The listing builds one solid part. Answer for the finished solid, in the listing's coordinates (mm). A direction names the side the tool comes from. Round coordinates to 2 decimals unless told otherwise and drop trailing zeros. Loops run counter-clockwise (first coordinate to the right, second up) from the corner with the lowest first, then second, coordinate; pieces in that order, holes last. Notation, with made-up numbers: (82.25, 41) -> (137.25, 41) arc R14 cw to (137.25, 56) -> close; hole circle Ø4 at (36, 63.5). An arc over 180 degrees is marked (long way). One line per question, with ' | ' between items.
from build123d import *

# Parameters (mm, degrees)
SKETCH_W             = 70
SKETCH_H             = 40
PAD_DEPTH            = 8.8
POCKET_DEPTH         = 4
SKETCH002_R          = 2
POCKET001_DEPTH      = 4.801
SKETCH003_W          = 64.25
SKETCH003_H          = 24
POCKET002_DEPTH      = 4.8
SKETCH004_R          = 2
POCKET003_DEPTH      = 4
SKETCH005_W          = 35
SKETCH005_H          = 12
POCKET004_DEPTH      = 4
POCKET005_DEPTH      = 8.801
SKETCH009_W          = 5.75
SKETCH009_H          = 15
POCKET006_DEPTH      = 2.3
FILLET_R             = 2.75
CHAMFER_SIZE         = 1
BODY_PLACEMENT_ANGLE = 90


with BuildPart() as part:
    # Sketch → Pad (new body)
    with BuildSketch(Plane.XZ):
        Rectangle(SKETCH_W, SKETCH_H)
    extrude(amount=PAD_DEPTH)

    # Sketch001 (on Face5 of Pad) → Pocket (cut)
    with BuildSketch(Plane(origin=(0, 0, 0), x_dir=(1, 0, 0), z_dir=(0, 1, 0))):
        with BuildLine():
            Line((31.8, -20), (31.8, -7))
            ThreePointArc((31.8, -7), (31.507107, -6.292893), (30.8, -6))
            Line((30.8, -6), (-9.2, -6))
            ThreePointArc((-9.2, -6), (-9.907107, -6.292893), (-10.2, -7))
            Line((-10.2, -7), (-10.2, -20))
            Line((-10.2, -20), (31.8, -20))
        make_face()
    extrude(amount=-POCKET_DEPTH, mode=Mode.SUBTRACT)

    # Sketch002 (on Face7 of Pocket) → Pocket001 (cut, through all)
    with BuildSketch(Plane(origin=(0, -4, 0), x_dir=(1, 0, 0), z_dir=(0, 1, 0))):
        with Locations((-4.825, -11.78)):
            Circle(SKETCH002_R)
        with Locations((26.425, -11.78)):
            Circle(SKETCH002_R)
    extrude(amount=-POCKET001_DEPTH, mode=Mode.SUBTRACT)

    # Sketch003 (on Face5 of Pocket001) → Pocket002 (cut)
    with BuildSketch(Plane.XZ.offset(8.8)):
        with Locations((-2.875, -8)):
            Rectangle(SKETCH003_W, SKETCH003_H)
    extrude(amount=-POCKET002_DEPTH, mode=Mode.SUBTRACT)

    # Sketch004 (on Face4 of Pocket002) → Pocket003 (cut)
    with BuildSketch(Plane.XZ.offset(4)):
        with Locations((14.9, -3.25)):
            Circle(SKETCH004_R)
        with Locations((-31.5, -6.25)):
            Circle(SKETCH004_R)
    extrude(amount=-POCKET003_DEPTH, mode=Mode.SUBTRACT)

    # Sketch005 (on Face4 of Pocket003) → Pocket004 (cut)
    with BuildSketch(Plane.XZ.offset(4)):
        with Locations((5.5, -14)):
            Rectangle(SKETCH005_W, SKETCH005_H)
    extrude(amount=-POCKET004_DEPTH, mode=Mode.SUBTRACT)

    # Sketch008 (on Face2 of Pocket004) → Pocket005 (cut, through all)
    with BuildSketch(Plane(origin=(0, 0, 0), x_dir=(1, 0, 0), z_dir=(0, 1, 0))):
        with BuildLine():
            ThreePointArc((-7.5, 6), (-4.5, 3), (-1.5, 6))
            Line((-1.5, 8), (-1.5, 6))
            Line((-7.5, 8), (-1.5, 8))
            Line((-7.5, 8), (-7.5, 6))
        make_face()
    extrude(amount=-POCKET005_DEPTH, mode=Mode.SUBTRACT)

    # Sketch009 (on Face6 of Pocket005) → Pocket006 (cut)
    with BuildSketch(Plane.XZ.offset(8.8)):
        with BuildLine():
            Line((-35, 4), (5, 4))
            Line((5, 4), (5, 8.5))
            ThreePointArc((5, 8.5), (4.707107, 9.207107), (4, 9.5))
            Line((4, 9.5), (-35, 9.5))
            Line((-35, 9.5), (-35, 4))
        make_face()
        with Locations((32.125, -12.5)):
            Rectangle(SKETCH009_W, SKETCH009_H)
    extrude(amount=-POCKET006_DEPTH, mode=Mode.SUBTRACT)

    # Fillet
    fillet_edges = [part.edges().sort_by_distance(p)[0] for p in [
        (35, -4.4, 20),
        (-35, -4.4, 20),
        (35, -3.25, -20),
        (-35, -2, -20),
    ]]
    fillet(fillet_edges, radius=FILLET_R)

    # Chamfer
    chamfer_edges = [part.edges().sort_by_distance(p)[0] for p in [
        (-10.2, -2, 20),
    ]]
    chamfer(chamfer_edges, length=CHAMFER_SIZE)


with BuildPart() as part_1:
    # Body placement: moved
    add(part.part.rotate(Axis((0, 0, 0), (-1, 0, 0)), BODY_PLACEMENT_ANGLE))


solid = part_1.part
Q1. For faces 1 (the face through (32, -12, 6.5)), 2 (the face through (-7.5, -7, 2)), 3 (the face through (10, 13, 4)), determine the directions among +Z, -Z, +X, -X, +Y, -Y from which every point of the face is accessible in a straight line to the end or side of a thin tool.
Numbers:
face 1: +Z, +X, -X, -Y | face 2: +Z, -Z, -Y | face 3: -Z, +Y
Q2. A cutting plane is placed at B-B on y = 11.78. Give the vertices of the cut face in (x, z) (3 decimals), plus the area to 3 significant figures.
Numbers:
outline: (-35, 0) -> (-10.2, 0) -> (-10.2, 4) -> (-6.825, 4) -> (-6.825, 8.8) -> (-35, 8.8) -> close; (-2.825, 4) -> (24.425, 4) -> (24.425, 8.8) -> (-2.825, 8.8) -> close; (28.425, 4) -> (31.8, 4) -> (31.8, 0) -> (35, 0) -> (35, 8.8) -> (28.425, 8.8) -> close | area: 410 mm^2
Q3. Given pin 1 Ø12 at (x, y) = (7.5, -9) entering from +Z; pin 2 Ø2.5 at (x, z) = (-14, 5.5) entering from -Y; pin 3 Ø3 at (x, z) = (13.5, 1) entering from -Y, each flat-ended and moving along its own axis, determine where each tip first touches the part or whether it passes through.
Numbers:
pin 1: z = 4 | pin 2: y = 4 | pin 3: y = -8
Q4. For a pull along X with two mould halves and no side action, classify faces 4 (the face through (-3, -2, 4)), 5 (the face through (-34.22, -19.17, 2.03)), 6 (the face through (-12, -14, 2)) as pulls with the +X half, pulls with the -X half, needs draft (parallel to the pull), parting line crosses it, or undercut.
Numbers:
face 4: needs draft | face 5: pulls with the -X half | face 6: undercut
Q5. A cutting plane is placed at D-D on z = 1.5. Give the vertices of the cut face in (x, y).
Numbers:
outline: (-35, -17.25) arc R2.75 ccw to (-32.25, -20) -> (-12, -20) -> (-12, -8) -> (-7.5, -8) -> (-7.5, -6) arc R3 cw to (-1.5, -6) -> (-1.5, -8) -> (23, -8) -> (23, -20) -> (32.25, -20) arc R2.75 ccw to (35, -17.25) -> (35, 17.25) arc R2.75 ccw to (32.25, 20) -> (31.8, 20) -> (31.8, 7) arc R1 cw to (30.8, 6) -> (-9.2, 6) arc R1 cw to (-10.2, 7) -> (-10.2, 19) -> (-11.2, 20) -> (-32.25, 20) arc R2.75 ccw to (-35, 17.25) -> close; hole circle Ø4 at (-31.5, -6.25); hole circle Ø4 at (14.9, -3.25)
Q6. A cutting plane is placed at C-C on x = -22. Give the vertices of the cut face in (y, z).
Numbers:
outline: (-20, 0) -> (20, 0) -> (20, 8.8) -> (9.5, 8.8) -> (9.5, 6.5) -> (4, 6.5) -> (4, 4) -> (-20, 4) -> close
Q7. A cutting plane is placed at A-A on x = 14.9. Give the vertices of the cut face in (y, z), plus the area to 3 significant figures.
Numbers:
outline: (-8, 0) -> (-5.25, 0) -> (-5.25, 4) -> (-8, 4) -> close; (-1.25, 0) -> (6, 0) -> (6, 4) -> (20, 4) -> (20, 8.8) -> (4, 8.8) -> (4, 4) -> (-1.25, 4) -> close | area: 117 mm^2
Q8. Find the intervals of material crossed by line 1 (X direction, y = -10.5, z = 0.5); line 2 (Y direction, x = 14.9, z = 2.3); line 3 (Y direction, x = -31.5, z = 1.45), in increasing order. Write a range as from..to.
Numbers:
line 1: -35..-12, 23..35 | line 2: -8..-5.25, -1.25..6 | line 3: -20..-8.25, -4.25..20
